Geometry check sheet. Reference: the model listing, model coordinates, mm. A direction names the side the tool comes from. Round coordinates to 2 decimals unless told otherwise and drop trailing zeros. Order: outer loops, then holes, each group sorted by start corner. A loop starts at its lowest first (then second) coordinate and runs counter-clockwise, first axis right, second up. Notation, with made-up numbers: (-18.5, 70) - (1.5, 70) arc R25 cw to (1.5, 84) - close; hole circle Ø7 at (61.5, 82.5). An arc over 180 degrees is marked (long way). One line per question, with ' | ' between items. Start each with the question number.
Q1. Material ranges on line 1 along X through (y, z) = (6, 1.05); line 2 along X through (y, z) = (-2.75, 1.4); line 3 along X through (y, z) = (1.25, 1.2), recorded low to high.
Q2. Sectioned sample at D-D, the plane x = -3. Enter the section's corners in (y, z), then the cut area to 3 significant figures.
Q3. Sectioned sample at B-B, the plane z = 1.15. Enter the section's corners in (x, y) (1 decimal), then the cut area to 3 significant figures.
Q4. Sectioned sample at C-C, the plane y = 8.25. Enter the section's corners in (x, z).
Q5. Gauge pin test, flat ends, axial feed: P1, Ø2, axis at x = 3.5, y = -0.5, coming from the -Z side; P2, Ø0.5, axis at y = 6.5, z = 1, coming from the -X side; P3, Ø1, axis at x = -0.5, y = 0, coming from the -Z side. Record the tip position at first contact, or that the pin passes through.
Q6. Mould release check, pull along X, two halves, no side actions. Record for faces 4 (the face through (0.22, 5.45, 1.511)), 5 (the face through (0, 3, 0)), 6 (the face through (0.805, 10.751, 0.783)): +X half, -X half, draft (parallel to the pull), parting line (faces both ways), or undercut.
Q7. Sectioned sample at A-A, the plane y = 0. Enter the section's corners in (x, z), then the cut area to 3 significant figures.
Q8. Tool access check on faces 1 (the face through (-0.159, -4.124, 0.783)), 2 (the face through (1.588, 6, 1)), 3 (the face through (-1.588, 6, 1)). Record the directions out of +Z, -Z, +X, -X, +Y, -Y that give a thin tool (end or side, any length) a straight path to the whole face; none if there is none.
```python
from build123d import *

# Parameters (mm, degrees)
SKETCH1_R           = 1.651
BOSS_EXTRUDE1_DEPTH = 1.5875
WRAP1_START         = -0.0762
WRAP1_DEPTH         = 0.0762


# Read off the part's stored shape, not the designer's step: Wrap1
with BuildPart() as part:
    # Sketch1 → Boss-Extrude1 (new body)
    with BuildSketch(Plane.XY):
        with BuildLine():
            Line((1.5875, 3.81), (1.5875, 7.62))
            Line((1.5875, 7.62), (0, 13.97))
            Line((0, 13.97), (-1.5875, 7.62))
            Line((-1.5875, 7.62), (-1.5875, 3.81))
            ThreePointArc((-1.5875, 3.81), (0, -4.1275), (1.5875, 3.81))
        make_face()
        Circle(SKETCH1_R, mode=Mode.SUBTRACT)
    extrude(amount=BOSS_EXTRUDE1_DEPTH)

    # Wrap1 outline → Wrap1 (cut)
    with BuildSketch(Plane.XY.offset(1.5875).offset(WRAP1_START)):
        with BuildLine():
            add(Edge.make_bspline(
                [(-0.6927271, 4.333675895), (-0.692495741, 4.33563577), (-0.691667591, 4.342651153), (-0.688769042, 4.357634786), (-0.684922586, 4.381892615), (-0.67986008, 4.412498716), (-0.674554045, 4.443717389), (-0.669757497, 4.46963377), (-0.666454834, 4.487377562), (-0.664707266, 4.496426288), (-0.664092904, 4.499607388)],
                knots=[0, 0, 0, 0, 0.035151439, 0.125824754, 0.271689381, 0.472746348, 0.678464873, 0.835817972, 0.942281445, 1, 1, 1, 1], degree=3))
            add(Edge.make_bspline(
                [(-0.51688377, 4.15746546), (-0.528701611, 4.158083472), (-0.551766092, 4.159289625), (-0.584872692, 4.169297645), (-0.615121792, 4.185426226), (-0.642244185, 4.207325789), (-0.664332359, 4.234330011), (-0.681129984, 4.264680596), (-0.690817492, 4.298344301), (-0.69208232, 4.321746179), (-0.6927271, 4.333675895)],
                knots=[0, 0, 0, 0, 0.127822844, 0.24946752, 0.37103994, 0.497334401, 0.624467945, 0.746667569, 0.870857209, 1, 1, 1, 1], degree=3))
            Line((-0.51688377, 4.15746546), (0.613065645, 4.15746546))
            add(Edge.make_bspline(
                [(0.619306431, 4.50841791), (0.632717748, 4.507153173), (0.658098658, 4.50475966), (0.693273978, 4.494445608), (0.722975165, 4.478932226), (0.747198284, 4.458294651), (0.765727881, 4.432501536), (0.778201608, 4.401557742), (0.784922795, 4.365808024), (0.785968558, 4.327125755), (0.782797594, 4.288646449), (0.774105079, 4.253571852), (0.760372999, 4.223441901), (0.740443682, 4.199291643), (0.716043821, 4.179781436), (0.685855522, 4.166902638), (0.65108202, 4.158569199), (0.62621445, 4.157847212), (0.613065645, 4.15746546)],
                knots=[0, 0, 0, 0, 0.072730168, 0.137641809, 0.196854627, 0.25270236, 0.308172367, 0.366921054, 0.43168746, 0.503873594, 0.5756551, 0.639861159, 0.698475495, 0.753049963, 0.807728666, 0.865787403, 0.929034673, 1, 1, 1, 1], degree=3))
            Line((0.619306431, 4.50841791), (-0.299924672, 4.50841791))
            add(Edge.make_bspline(
                [(-0.265416795, 4.61340996), (-0.266287441, 4.611335244), (-0.268671287, 4.605654632), (-0.272648022, 4.594488112), (-0.278056178, 4.578425355), (-0.284599105, 4.559148006), (-0.290437621, 4.540090467), (-0.295453112, 4.524748532), (-0.298353833, 4.514818948), (-0.299563911, 4.509887977), (-0.299924672, 4.50841791)],
                knots=[0, 0, 0, 0, 0.061041746, 0.16713346, 0.321479673, 0.520970162, 0.719435699, 0.862244331, 0.958930983, 1, 1, 1, 1], degree=3))
            add(Edge.make_bspline(
                [(0.027165948, 5.075595247), (0.012329066, 5.058837564), (-0.017572968, 5.025064378), (-0.06002472, 4.971553167), (-0.101552202, 4.915829097), (-0.141371923, 4.857947546), (-0.178311252, 4.798326659), (-0.211983981, 4.737785905), (-0.241000061, 4.676139025), (-0.257329382, 4.634187343), (-0.265416795, 4.61340996)],
                knots=[0, 0, 0, 0, 0.12202016, 0.245917621, 0.372291213, 0.500915216, 0.628859031, 0.754584526, 0.878453238, 1, 1, 1, 1], degree=3))
            add(Edge.make_bspline(
                [(0.391334181, 5.361937204), (0.361223865, 5.337586417), (0.300850401, 5.288761242), (0.219924135, 5.235074247), (0.155397551, 5.192066323), (0.110122794, 5.155965467), (0.066910538, 5.117642292), (0.040427943, 5.089625526), (0.027165948, 5.075595247)],
                knots=[0, 0, 0, 0, 0.250087632, 0.501444657, 0.627123169, 0.750990091, 0.875300439, 1, 1, 1, 1], degree=3))
            add(Edge.make_bspline(
                [(0.598381442, 5.56494631), (0.581926642, 5.547262699), (0.549082849, 5.511966198), (0.49868679, 5.460177761), (0.447122843, 5.409034831), (0.410033576, 5.377723514), (0.391334181, 5.361937204)],
                knots=[0, 0, 0, 0, 0.249702456, 0.49840631, 0.747110164, 1, 1, 1, 1], degree=3))
            add(Edge.make_bspline(
                [(0.33920526, 6.656716797), (0.353472465, 6.651511564), (0.381587775, 6.641254003), (0.421878928, 6.623018524), (0.46040127, 6.60379966), (0.496246373, 6.581804576), (0.530707302, 6.55893057), (0.562434404, 6.533414044), (0.592544673, 6.506642148), (0.619896671, 6.477556983), (0.645403722, 6.446910926), (0.668952012, 6.414618565), (0.690309115, 6.380391375), (0.709306159, 6.344213139), (0.726787061, 6.306508462), (0.741234339, 6.266585002), (0.754241409, 6.22511982), (0.768072724, 6.168006218), (0.780178454, 6.096569678), (0.784368607, 6.011894186), (0.778401012, 5.930079625), (0.763237068, 5.850700165), (0.736754159, 5.774454593), (0.700650258, 5.70108113), (0.65499011, 5.630171698), (0.617543834, 5.587025516), (0.598381442, 5.56494631)],
                knots=[0, 0, 0, 0, 0.034109449, 0.067216932, 0.099308832, 0.130758354, 0.161641564, 0.192170293, 0.22214936, 0.252098155, 0.281773115, 0.311689081, 0.341822813, 0.372324293, 0.403451297, 0.435115199, 0.467638762, 0.501046257, 0.567081754, 0.630114049, 0.691033314, 0.750991448, 0.811157234, 0.871775484, 0.934383635, 1, 1, 1, 1], degree=3))
            add(Edge.make_bspline(
                [(-0.538910074, 6.14387101), (-0.533666781, 6.168600667), (-0.523379004, 6.217122316), (-0.49947922, 6.286622214), (-0.46952229, 6.351736346), (-0.432141963, 6.411594101), (-0.388817022, 6.467103624), (-0.338443531, 6.517468922), (-0.281818221, 6.563499117), (-0.219357577, 6.603751762), (-0.153537671, 6.638071584), (-0.085716569, 6.665195555), (-0.016745257, 6.684019917), (0.053090433, 6.694810558), (0.123668827, 6.69725602), (0.195052802, 6.69205738), (0.26744334, 6.678845403), (0.314983363, 6.664185895), (0.33920526, 6.656716797)],
                knots=[0, 0, 0, 0, 0.065457993, 0.128434036, 0.190005232, 0.250812254, 0.310887235, 0.372102182, 0.434999136, 0.499647143, 0.564322364, 0.62709449, 0.688559438, 0.749194229, 0.80980248, 0.871165092, 0.934357921, 1, 1, 1, 1], degree=3))
            add(Edge.make_bspline(
                [(-0.54515086, 5.957748738), (-0.545718168, 5.961046078), (-0.547345693, 5.970505669), (-0.546773291, 5.989222056), (-0.547292664, 6.016483915), (-0.545797464, 6.049530152), (-0.544775877, 6.082836829), (-0.54278109, 6.110594522), (-0.541383604, 6.130127097), (-0.539569617, 6.140206325), (-0.538910074, 6.14387101)],
                knots=[0, 0, 0, 0, 0.053703755, 0.154068263, 0.299667211, 0.492577764, 0.685558541, 0.835415856, 0.940159201, 1, 1, 1, 1], degree=3))
            add(Edge.make_bspline(
                [(-0.313507559, 5.817881705), (-0.326748688, 5.814308009), (-0.352565283, 5.807340274), (-0.392277197, 5.807775651), (-0.430582168, 5.815853055), (-0.465914446, 5.832877527), (-0.497319983, 5.855880409), (-0.521377363, 5.885403501), (-0.538261794, 5.91971928), (-0.542813227, 5.944844385), (-0.54515086, 5.957748738)],
                knots=[0, 0, 0, 0, 0.132186122, 0.257726952, 0.380150903, 0.508367113, 0.634381904, 0.753877808, 0.873590673, 1, 1, 1, 1], degree=3))
            add(Edge.make_bspline(
                [(-0.198236566, 5.998864506), (-0.197479077, 5.989433957), (-0.195955535, 5.970466259), (-0.200815888, 5.941934255), (-0.210542191, 5.913916125), (-0.225203232, 5.887363551), (-0.242888924, 5.862861999), (-0.264463419, 5.843302102), (-0.287482268, 5.827105268), (-0.304880803, 5.820939094), (-0.313507559, 5.817881705)],
                knots=[0, 0, 0, 0, 0.122295461, 0.245973298, 0.371951377, 0.505452265, 0.638129912, 0.761654916, 0.881820808, 1, 1, 1, 1], degree=3))
            add(Edge.make_bspline(
                [(-0.199704987, 6.015017129), (-0.199566206, 6.013672938), (-0.199276128, 6.010863318), (-0.199164855, 6.006656873), (-0.198039254, 6.00269879), (-0.198173285, 6.000094218), (-0.198236566, 5.998864506)],
                knots=[0, 0, 0, 0, 0.249515153, 0.521535263, 0.774099595, 1, 1, 1, 1], degree=3))
            add(Edge.make_bspline(
                [(0.285975025, 6.294751195), (0.272682151, 6.302411025), (0.246820565, 6.317313396), (0.206070499, 6.333889959), (0.164895436, 6.343180125), (0.123783852, 6.347764309), (0.082451701, 6.344774208), (0.040930466, 6.336302375), (-0.000789689, 6.321390173), (-0.041463496, 6.300532784), (-0.079886926, 6.276014174), (-0.113287346, 6.247194805), (-0.142021611, 6.216160745), (-0.164514541, 6.181366891), (-0.182237478, 6.144073312), (-0.193171755, 6.103402582), (-0.200370718, 6.060183865), (-0.199930896, 6.03034404), (-0.199704987, 6.015017129)],
                knots=[0, 0, 0, 0, 0.066639456, 0.12964856, 0.190280739, 0.249604232, 0.308755828, 0.369565023, 0.433317181, 0.500628138, 0.567894957, 0.630888346, 0.691885636, 0.751037232, 0.810284388, 0.870553939, 0.933511396, 1, 1, 1, 1], degree=3))
            add(Edge.make_bspline(
                [(0.343243416, 5.806868553), (0.351118523, 5.816407152), (0.366580785, 5.835135574), (0.386597777, 5.865012057), (0.402782369, 5.896097243), (0.415819128, 5.928119207), (0.424960671, 5.961266887), (0.430570708, 5.995358807), (0.432217895, 6.030307207), (0.430871446, 6.06572163), (0.425827166, 6.10070134), (0.417013572, 6.134350041), (0.404442271, 6.166146407), (0.388279505, 6.196056065), (0.368152112, 6.223808343), (0.34445221, 6.249741409), (0.316833874, 6.273573162), (0.296395252, 6.287599927), (0.285975025, 6.294751195)],
                knots=[0, 0, 0, 0, 0.065983685, 0.129554698, 0.191477678, 0.252715103, 0.313711813, 0.374582555, 0.43670492, 0.500101288, 0.563453918, 0.624910304, 0.685299263, 0.74549372, 0.805843828, 0.867780579, 0.932590547, 1, 1, 1, 1], degree=3))
            add(Edge.make_bspline(
                [(0.023494898, 5.525298962), (0.053077007, 5.546024218), (0.110773274, 5.586446284), (0.191248753, 5.654420756), (0.268021717, 5.7279068), (0.317633659, 5.779985467), (0.343243416, 5.806868553)],
                knots=[0, 0, 0, 0, 0.25365197, 0.494716981, 0.739172156, 1, 1, 1, 1], degree=3))
            add(Edge.make_bspline(
                [(-0.664092904, 4.499607388), (-0.658464763, 4.524753093), (-0.647193012, 4.575113612), (-0.625796845, 4.649765684), (-0.600307799, 4.723379254), (-0.571857224, 4.796338257), (-0.538895385, 4.867967849), (-0.502663605, 4.938847518), (-0.462420857, 5.008682301), (-0.419106564, 5.077470685), (-0.372126214, 5.143890883), (-0.323106184, 5.207984837), (-0.27111994, 5.26850968), (-0.217145112, 5.326365759), (-0.160639031, 5.380988853), (-0.101805622, 5.43256559), (-0.040448995, 5.480747144), (0.002179636, 5.510447916), (0.023494898, 5.525298962)],
                knots=[0, 0, 0, 0, 0.061108243, 0.122384435, 0.184064158, 0.245829863, 0.308042655, 0.37099844, 0.434574042, 0.499151414, 0.563730742, 0.627472417, 0.690465657, 0.752889321, 0.815082475, 0.876788142, 0.938391336, 1, 1, 1, 1], degree=3))
        make_face()
    extrude(amount=WRAP1_DEPTH, mode=Mode.SUBTRACT)


solid = part.part
```
Determined:
1) line 1: x = -1.59 to 1.59 | line 2: x = -3.08 to 3.08 | line 3: x = -3.93 to -1.08, 1.08 to 3.93
2) outline: (-2.83, 0) - (2.83, 0) - (2.83, 1.59) - (-2.83, 1.59) - close | area: 9.00 mm2
3) outline: (-1.6, 3.8) arc R4.1 ccw (long way) to (1.6, 3.8) - (1.6, 7.6) - (0, 14) - (-1.6, 7.6) - close; hole circle Ø3.3 at (0, 0) | area: 66.5 mm2
4) outline: (-1.43, 0) - (1.43, 0) - (1.43, 1.59) - (-1.43, 1.59) - close
5) P1: stops at z = 0 | P2: stops at x = -1.59 | P3: passes through
6) face 4: undercut | face 5: draft | face 6: +X half
7) outline: (-4.13, 0) - (-1.65, 0) - (-1.65, 1.59) - (-4.13, 1.59) - close; (1.65, 0) - (4.13, 0) - (4.13, 1.59) - (1.65, 1.59) - close | area: 7.86 mm2
8) face 1: +Z, -Z | face 2: +Z, -Z, +X, +Y | face 3: +Z, -Z, -X, +Y
